The listing builds one solid part. Answer for the finished solid, in the listing's coordinates (mm). Face numbers are marked on the shaded views. A direction names the side the tool comes from. Coordinates: 2 decimals unless noted, no trailing zeros. Order: outer loops, then holes, each group sorted by start corner. A loop starts at its lowest first (then second) coordinate and runs counter-clockwise, first axis right, second up. Notation, with made-up numbers: (7.25, -37) -> (61.25, -37) arc R20 ccw to (61.25, -25) -> close; hole circle Ø11 at (79.5, 72). An arc over 180 degrees is marked (long way). Answer in a Markdown table with one row per item.
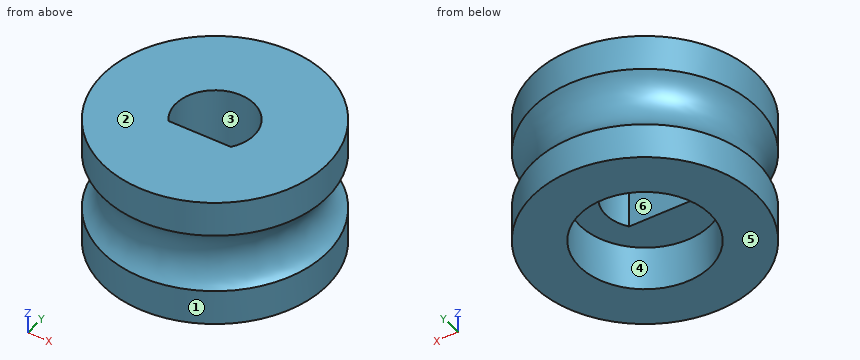
```python
from build123d import *

# Parameters (mm, degrees)
SKETCH_R     = 3
PAD_DEPTH    = 3.5
SKETCH002_R  = 1.75
POCKET_DEPTH = 1.2
TORUS_R      = 1


with BuildPart() as part:
    # Sketch → Pad (new body)
    with BuildSketch(Plane.XY):
        Circle(SKETCH_R)
        with BuildLine():
            ThreePointArc((0.843727, -0.625), (0, 1.05), (-0.843727, -0.625))
            Line((-0.843727, -0.625), (0.843727, -0.625))
        make_face(mode=Mode.SUBTRACT)
    extrude(amount=PAD_DEPTH)

    # Sketch002 (on Face4 of Pad) → Pocket (cut)
    with BuildSketch(Plane(origin=(0, 0, 0), x_dir=(1, 0, 0), z_dir=(0, 0, -1))):
        Circle(SKETCH002_R)
    extrude(amount=-POCKET_DEPTH, mode=Mode.SUBTRACT)

    # Torus → Torus (revolve, cut)
    with BuildSketch(Plane(origin=(0, 0, 1.75), x_dir=(1, 0, 0), z_dir=(0, -1, 0))):
        with Locations((3.6, 0)):
            Circle(TORUS_R)
    revolve(axis=Axis((0, 0, 1.75), (0, 0, 1)), mode=Mode.SUBTRACT)


solid = part.part
```
(1) Which of the six approach directions +Z, -Z, +X, -X, +Y, -Y give full straight-line access (tool end or side, diameter ignored) to the marked faces 4, 5 and 6?
Check values:
| item | result |
|---|---|
| face 4 | -Z |
| face 5 | -Z, +X, -X, +Y, -Y |
| face 6 | +Z, -Z |
(2) For a pull along Y with two mould halves and no side action, classify the marked faces 1, 2 and 3 as released by +Y, released by -Y, zero draft, split by the parting line, or undercut.
Check values:
| item | result |
|---|---|
| face 1 | split by the parting line |
| face 2 | zero draft |
| face 3 | undercut |
(3) Find the intervals of material crossed by line 1 along Y through (x, z) = (0, 3) (3 decimals); line 2 along Y through (x, z) = (0, 0.6); line 3 along Z through (x, y) = (0.25, 1.6), in increasing order. Write a range as from..to.
Check values:
| item | result |
|---|---|
| line 1 | -3..-0.625, 1.05..3 |
| line 2 | -3..-1.75, 1.75..3 |
| line 3 | 1.2..3.5 |
(4) A cutting plane is placed at B-B, the plane z = 2.95. Determine the outline of the cut face in (x, y) (3 decimals).
Check values:
| item | result |
|---|---|
| outline | circle Ø6 at (0, 0); hole (-0.844, -0.625) -> (0.844, -0.625) arc R1.05 ccw (long way) to start |
(5) A cutting plane is placed at A-A, the plane y = 0. Determine the outline of the cut face in (x, z), then the cut area to 3 significant figures.
Check values:
| item | result |
|---|---|
| outline | (-3, 0) -> (-1.75, 0) -> (-1.75, 1.2) -> (-1.05, 1.2) -> (-1.05, 3.5) -> (-3, 3.5) -> (-3, 2.55) arc R1 cw to (-3, 0.95) -> close; (1.05, 1.2) -> (1.75, 1.2) -> (1.75, 0) -> (3, 0) -> (3, 0.95) arc R1 cw to (3, 2.55) -> (3, 3.5) -> (1.05, 3.5) -> close |
| area | 11.1 mm² |
(6) Flat-ended cylindrical pins translate along their axes: pin 1 (1.5 mm diameter, centred on x = 2, z = 0.5, fed in from -Y); pin 2 (2.5 mm diameter, centred on x = 0, y = 0, fed in from -Z); pin 3 (0.5 mm diameter, centred on x = -0.5, z = 2, fed in from +Y). Find the tip coordinate at first contact, or state that the pin passes through.
Check values:
| item | result |
|---|---|
| pin 1 | y = -2.73 |
| pin 2 | z = 1.2 |
| pin 3 | y = 2.69 |
